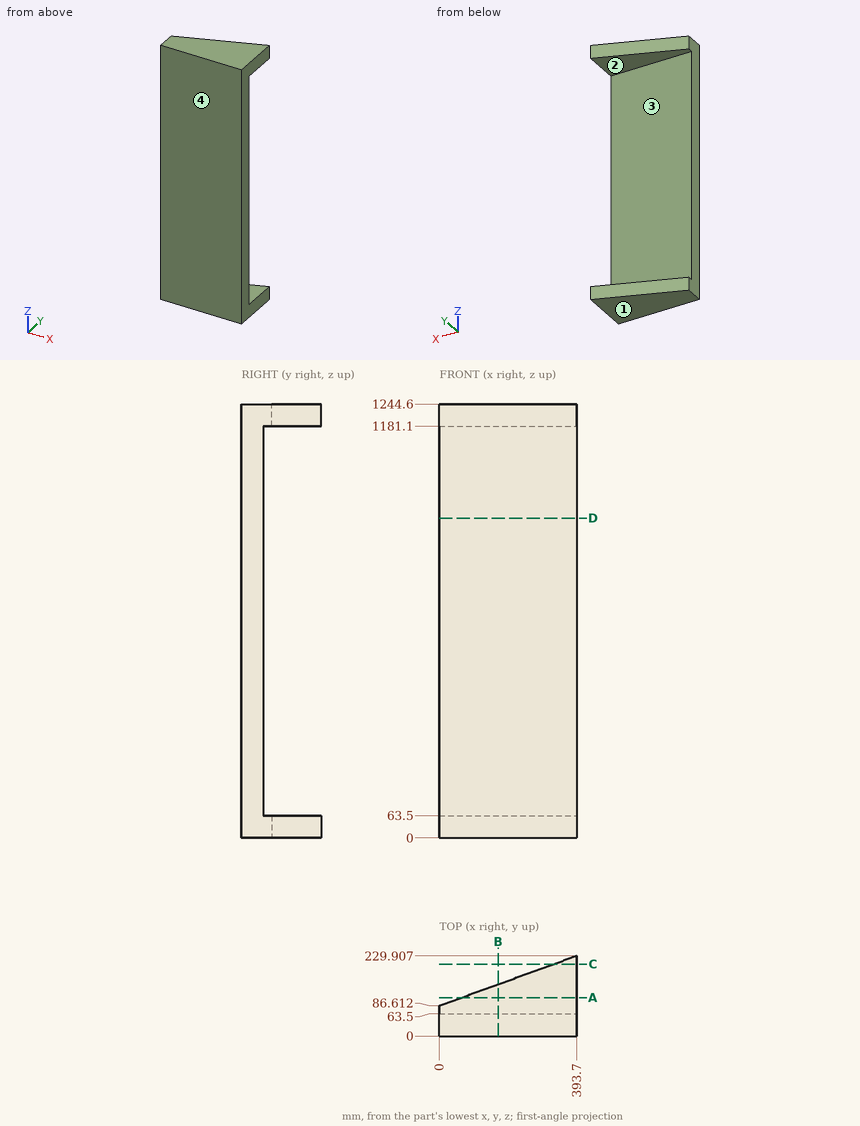
Drawing for the job (mm, zero at the part's lowest x, y, z). Round coordinates to 2 decimals unless told otherwise and drop trailing zeros. Order: outer loops, then holes, each group sorted by start corner. A loop starts at its lowest first (then second) coordinate and runs counter-clockwise, first axis right, second up. Notation, with made-up numbers: M 59.5,60 L 76.5,60 A21 ccw 76.5,73 Z; hole C -13,76 d1. An arc over 180 degrees is marked long. Use one line per item in the form item = value.
Q1. Flat gauge pin, fed straight in: P1, Ø2, axis at x = 99, z = 983.5, coming from the +Y side. Where does the tip first touch, or does it go through?
Recorded:
P1 = 63.5
Q2. Saw through at C-C on y = 206.5. Give the cut face in (x, z), then the cut area to 3 significant figures.
Recorded:
outline = M 329.39,0 L 393.7,0 L 393.7,63.5 L 329.39,63.5 Z; M 329.39,1181.1 L 393.7,1181.1 L 393.7,1244.6 L 329.39,1244.6 Z
area = 8,170 mm^2
Q3. Saw through at B-B on x = 168. Give the cut face in (y, z).
Recorded:
outline = M 0,0 L 147.76,0 L 147.76,63.5 L 63.5,63.5 L 63.5,1181.1 L 147.76,1181.1 L 147.76,1244.6 L 0,1244.6 Z
Q4. Two-plate mould, pull along Z, no slides. Class the marked faces 1, 2, 3 and 4: +Z half, -Z half, draft (parallel to the pull), parting line (faces both ways), or undercut.
Recorded:
face_1 = -Z half
face_2 = undercut
face_3 = undercut
face_4 = draft
Q5. Saw through at A-A on y = 110. Give the cut face in (x, z), then the cut area to 3 significant figures.
Recorded:
outline = M 64.26,0 L 393.7,0 L 393.7,63.5 L 64.26,63.5 Z; M 64.26,1181.1 L 393.7,1181.1 L 393.7,1244.6 L 64.26,1244.6 Z
area = 41,800 mm^2
Q6. Saw through at D-D on z = 917.5. Give the cut face in (x, y), then the cut area to 3 significant figures.
Recorded:
outline = M 0,0 L 393.7,0 L 393.7,63.5 L 0,63.5 Z
area = 25,000 mm^2
Q7. Probe L1, parallel to Z at x = 193, y = 117; L2, parallel to Y at x = 338.5, z = 711.5. List the from-to ranges inside material, lowest first.
Recorded:
L1 = 0 to 63.5, 1181.1 to 1244.6
L2 = 0 to 63.5
